Geometry check sheet. Reference: the model listing, model coordinates, mm. A direction names the side the tool comes from. Give positions to 0.01 mm unless a question says otherwise; leave off trailing zeros. Order: outer loops, then holes, each group sorted by start corner. A loop starts at its lowest first (then second) coordinate and runs counter-clockwise, first axis right, second up.
```python
from build123d import *

# Parameters (mm, degrees)
EXTRUDE_START          = 0.5
EXTRUDE_0_5_1_2_DEPTH  = 1.2
EXTRUDE_1_7_DEPTH      = 1.7
EXTRUDE_START_2        = 1.7
SKETCH_721_R           = 1.9
EXTRUDE_774_DEPTH      = 0.9373
SKETCH_M2_R            = 1.1
CUT_EXTRUDE_907_DEPTH  = 28.562571565
SKETCH_M3_R            = 1.7
CUT_EXTRUDE_1008_DEPTH = 28.562571565
CUT_EXTRUDE_1244_DEPTH = 28.562571565
CHAMFER_C0_15_SIZE     = 0.15


with BuildPart() as part:
    # Sketch 220 → 托板抬高0_5并厚1_2 (new body)
    with BuildSketch(Plane.XY.offset(EXTRUDE_START)):
        with BuildLine():
            Line((-12.4, -15.7), (12.4, -15.7))
            ThreePointArc((12.4, -15.7), (13.460660172, -15.260660172), (13.9, -14.2))
            Line((13.9, -14.2), (13.9, 0.8))
            ThreePointArc((13.9, 0.8), (13.460660172, 1.860660172), (12.4, 2.3))
            Line((12.4, 2.3), (-12.4, 2.3))
            ThreePointArc((-12.4, 2.3), (-13.460660172, 1.860660172), (-13.9, 0.8))
            Line((-13.9, 0.8), (-13.9, -14.2))
            ThreePointArc((-13.9, -14.2), (-13.460660172, -15.260660172), (-12.4, -15.7))
        make_face()
        with BuildLine():
            Line((-7, -12.2), (7, -12.2))
            ThreePointArc((7, -12.2), (7.707106781, -11.907106781), (8, -11.2))
            Line((8, -11.2), (8, -1.2))
            ThreePointArc((8, -1.2), (7.707106781, -0.492893219), (7, -0.2))
            Line((7, -0.2), (-7, -0.2))
            ThreePointArc((-7, -0.2), (-7.707106781, -0.492893219), (-8, -1.2))
            Line((-8, -1.2), (-8, -11.2))
            ThreePointArc((-8, -11.2), (-7.707106781, -11.907106781), (-7, -12.2))
        make_face(mode=Mode.SUBTRACT)
    extrude(amount=EXTRUDE_0_5_1_2_DEPTH)

    # Sketch 459 → 安装耳底面基准与厚1_7 (add)
    with BuildSketch(Plane.XY):
        with BuildLine():
            Line((-20.5, -8.5), (-12.5, -8.5))
            ThreePointArc((-12.5, -8.5), (-11.085786438, -7.914213562), (-10.5, -6.5))
            Line((-10.5, -6.5), (-10.5, -3.5))
            ThreePointArc((-10.5, -3.5), (-11.085786438, -2.085786438), (-12.5, -1.5))
            Line((-12.5, -1.5), (-20.5, -1.5))
            ThreePointArc((-20.5, -1.5), (-21.914213562, -2.085786438), (-22.5, -3.5))
            Line((-22.5, -3.5), (-22.5, -6.5))
            ThreePointArc((-22.5, -6.5), (-21.914213562, -7.914213562), (-20.5, -8.5))
        make_face()
        with BuildLine():
            Line((12.5, -8.5), (20.5, -8.5))
            ThreePointArc((20.5, -8.5), (21.914213562, -7.914213562), (22.5, -6.5))
            Line((22.5, -6.5), (22.5, -3.5))
            ThreePointArc((22.5, -3.5), (21.914213562, -2.085786438), (20.5, -1.5))
            Line((20.5, -1.5), (12.5, -1.5))
            ThreePointArc((12.5, -1.5), (11.085786438, -2.085786438), (10.5, -3.5))
            Line((10.5, -3.5), (10.5, -6.5))
            ThreePointArc((10.5, -6.5), (11.085786438, -7.914213562), (12.5, -8.5))
        make_face()
    extrude(amount=EXTRUDE_1_7_DEPTH)

    # Sketch 721 → Extrude 774 (add)
    with BuildSketch(Plane.XY.offset(EXTRUDE_START_2)):
        with Locations((-10.5, -12.4)):
            Circle(SKETCH_721_R)
        with Locations((-10.5, 0.1)):
            Circle(SKETCH_721_R)
        with Locations((10.5, -12.4)):
            Circle(SKETCH_721_R)
        with Locations((10.5, 0.1)):
            Circle(SKETCH_721_R)
    extrude(amount=EXTRUDE_774_DEPTH)

    # 四个相机M2间隙孔 → Cut-Extrude 907 (cut, through all)
    with BuildSketch(Plane.XY):
        with Locations((-10.5, -12.4)):
            Circle(SKETCH_M2_R)
        with Locations((-10.5, 0.1)):
            Circle(SKETCH_M2_R)
        with Locations((10.5, -12.4)):
            Circle(SKETCH_M2_R)
        with Locations((10.5, 0.1)):
            Circle(SKETCH_M2_R)
    extrude(amount=CUT_EXTRUDE_907_DEPTH, mode=Mode.SUBTRACT)

    # 双耳M3间隙孔 → Cut-Extrude 1008 (cut, through all)
    with BuildSketch(Plane.XY):
        with Locations((-20, -5)):
            Circle(SKETCH_M3_R)
        with Locations((20, -5)):
            Circle(SKETCH_M3_R)
    extrude(amount=CUT_EXTRUDE_1008_DEPTH, mode=Mode.SUBTRACT)

    # Sketch 1078 → Cut-Extrude 1244 (cut, through all)
    with BuildSketch(Plane.XY):
        with BuildLine():
            Line((7.2, -6.7), (10.2, -6.7))
            ThreePointArc((10.2, -6.7), (10.624264069, -6.524264069), (10.8, -6.1))
            Line((10.8, -6.1), (10.8, -3.1))
            ThreePointArc((10.8, -3.1), (10.624264069, -2.675735931), (10.2, -2.5))
            Line((10.2, -2.5), (7.2, -2.5))
            ThreePointArc((7.2, -2.5), (6.775735931, -2.675735931), (6.6, -3.1))
            Line((6.6, -3.1), (6.6, -6.1))
            ThreePointArc((6.6, -6.1), (6.775735931, -6.524264069), (7.2, -6.7))
        make_face()
        with BuildLine():
            Line((-10.2, -8.1), (-7.2, -8.1))
            ThreePointArc((-7.2, -8.1), (-6.775735931, -7.924264069), (-6.6, -7.5))
            Line((-6.6, -7.5), (-6.6, -4.5))
            ThreePointArc((-6.6, -4.5), (-6.775735931, -4.075735931), (-7.2, -3.9))
            Line((-7.2, -3.9), (-10.2, -3.9))
            ThreePointArc((-10.2, -3.9), (-10.624264069, -4.075735931), (-10.8, -4.5))
            Line((-10.8, -4.5), (-10.8, -7.5))
            ThreePointArc((-10.8, -7.5), (-10.624264069, -7.924264069), (-10.2, -8.1))
        make_face()
    extrude(amount=CUT_EXTRUDE_1244_DEPTH, mode=Mode.SUBTRACT)

    # 安装耳外缘去锐C0_15
    chamfer_c0_15_edges = [part.edges().sort_by_distance(p)[0] for p in [
        (21.914213562, -2.085786438, 1.7),
        (22.5, -5, 1.7),
        (21.914213562, -7.914213562, 1.7),
        (-21.914213562, -7.914213562, 1.7),
        (-21.914213562, -2.085786438, 1.7),
        (-22.5, -5, 1.7),
    ]]
    chamfer(chamfer_c0_15_edges, length=CHAMFER_C0_15_SIZE)


solid = part.part
```
Q1. Cross-section at C-C, the plane y = -9. Record the boundary of the cut face in (x, z).
Q2. Release check for a two-part mould opening along Y. For faces 4 (the face through (21.93, -2.1, 0.76)), 5 (the face through (13.9, 0, 1)), 6 (the face through (11.516, -0.321, 1.554)) record: pulls with the +Y half, pulls with the -Y half, needs draft (parallel to the pull), parting line crosses it, or undercut.
Q3. Cross-section at D-D, the plane x = -17. Record the boundary of the cut face in (y, z).
Q4. Cross-section at A-A, the plane z = 2.15. Record the boundary of the cut face in (x, y), and give its area (3 significant figures).
Q5. Access from +Z, -Z, +X, -X, +Y, -Y to the whole of each face (thin tool, end or side, straight path). Record for faces 1 (the face through (-13.47, -15.25, 1.09)), 2 (the face through (-9, -3.9, 1)), 3 (the face through (12.255, -0.628, 2.162)).
Q6. Cross-section at B-B, the plane x = -5.5. Record the boundary of the cut face in (y, z), and give its area (3 significant figures).
Q7. Thickness scan on L1, parallel to X at y = -12.4, z = 0.9; L2, parallel to Y at x = 10.5, z = 1.9; L3, parallel to X at y = -5, z = 1. Record the ranges inside material, lowest first.
Q8. Gauge pin test, flat ends, axial feed: P1, Ø1.3, axis at y = -2, z = 1, coming from the -X side; P2, Ø1, axis at y = 0, z = 1, coming from the +X side; P3, Ø0.8, axis at x = 15, z = 0.5, coming from the +Y side; P4, Ø2.5, axis at x = 4, y = -10, coming from the -Z side. Record the tip position at first contact, or that the pin passes through.
Answers follow:
1. outline: (-13.9, 0.5) - (-8, 0.5) - (-8, 1.7) - (-13.9, 1.7) - close; (8, 0.5) - (13.9, 0.5) - (13.9, 1.7) - (8, 1.7) - close
2. face 4: pulls with the +Y half
2. face 5: needs draft
2. face 6: undercut
3. outline: (-8.5, 0) - (-1.5, 0) - (-1.5, 1.55) - (-1.65, 1.7) - (-8.35, 1.7) - (-8.5, 1.55) - close
4. outline: circle Ø3.8 at (-10.5, -12.4); circle Ø3.8 at (-10.5, 0.1); circle Ø3.8 at (10.5, -12.4); circle Ø3.8 at (10.5, 0.1); hole circle Ø2.2 at (-10.5, -12.4); hole circle Ø2.2 at (-10.5, 0.1); hole circle Ø2.2 at (10.5, -12.4); hole circle Ø2.2 at (10.5, 0.1)
4. area: 30.2 mm2
5. face 1: +Z, -Z, -X, -Y
5. face 2: +Z, -Z
5. face 3: +Z
6. outline: (-15.7, 0.5) - (-12.2, 0.5) - (-12.2, 1.7) - (-15.7, 1.7) - close; (-0.2, 0.5) - (2.3, 0.5) - (2.3, 1.7) - (-0.2, 1.7) - close
6. area: 7.20 mm2
7. L1: x = -13.9 to -11.6, -9.4 to 9.4, 11.6 to 13.9
7. L2: y = -14.3 to -13.5, -11.3 to -10.5, -1.8 to -1, 1.2 to 2
7. L3: x = -22.5 to -21.7, -18.3 to -10.8, 10.8 to 18.3, 21.7 to 22.5
8. P1: stops at x = -22.31
8. P2: stops at x = 13.9
8. P3: stops at y = -1.5
8. P4: passes through
